```python
from build123d import *

# Parameters (mm, degrees)
BOSS_EXTRUDE1_DEPTH            = 4
CBORE_FOR_M3_SHCS2_D           = 3.4
CBORE_FOR_M3_SHCS2_CBORE_D     = 6.5
CBORE_FOR_M3_SHCS2_CBORE_DEPTH = 3
M5X0_8_TAPPED_HOLE1_D          = 4.2
M5X0_8_TAPPED_HOLE2_D          = 4.2
SKETCH8_W                      = 20
SKETCH8_H                      = 10
CUT_EXTRUDE1_DEPTH             = 5


with BuildPart() as part:
    # Sketch1 → Boss-Extrude1 (new body, symmetric)
    with BuildSketch(Plane.XY):
        with BuildLine():
            Line((-34.5, 0), (-49.5, 0))
            Line((-49.5, 0), (-49.5, 60))
            Line((-49.5, 60), (49.5, 60))
            Line((49.5, 60), (49.5, 0))
            Line((49.5, 0), (34.5, 0))
            Line((34.5, 0), (34.5, 47.5))
            ThreePointArc((34.5, 47.5), (33.767766953, 49.267766953), (32, 50))
            Line((32, 50), (-32, 50))
            ThreePointArc((-32, 50), (-33.767766953, 49.267766953), (-34.5, 47.5))
            Line((-34.5, 47.5), (-34.5, 0))
        make_face()
    extrude(amount=BOSS_EXTRUDE1_DEPTH, both=True)

    # CBORE for M3 SHCS2 (through all)
    with Locations(Plane.XY.offset(4)):
        with Locations((-42, 40), (-42, 20)):
            cbore_for_m3_shcs2 = CounterBoreHole(CBORE_FOR_M3_SHCS2_D / 2, CBORE_FOR_M3_SHCS2_CBORE_D / 2, CBORE_FOR_M3_SHCS2_CBORE_DEPTH)

    # M5x0.8 Tapped Hole1 (through all)
    with Locations(Plane.XY.offset(4)):
        with Locations((-42, 10), (-42, 50)):
            m5x0_8_tapped_hole1 = Hole(M5X0_8_TAPPED_HOLE1_D / 2)

    # M5x0.8 Tapped Hole2 (through all)
    with Locations(Plane(origin=(0, 60, 0), x_dir=(1, 0, 0), z_dir=(0, 1, 0))):
        with Locations((-28.5, 0)):
            m5x0_8_tapped_hole2 = Hole(M5X0_8_TAPPED_HOLE2_D / 2)

    # Mirror1: CBORE for M3 SHCS2, M5x0.8 Tapped Hole1, M5x0.8 Tapped Hole2 across plane
    add(cbore_for_m3_shcs2.mirror(Plane(origin=(0, 0, 0), x_dir=(0, 0, 1), z_dir=(1, 0, 0))), mode=Mode.SUBTRACT)
    add(m5x0_8_tapped_hole1.mirror(Plane(origin=(0, 0, 0), x_dir=(0, 0, 1), z_dir=(1, 0, 0))), mode=Mode.SUBTRACT)
    add(m5x0_8_tapped_hole2.mirror(Plane(origin=(0, 0, 0), x_dir=(0, 0, 1), z_dir=(1, 0, 0))), mode=Mode.SUBTRACT)

    # Sketch8 → Cut-Extrude1 (cut)
    with BuildSketch(Plane.XY.offset(4)):
        with Locations((0, 55)):
            Rectangle(SKETCH8_W, SKETCH8_H)
    extrude(amount=-CUT_EXTRUDE1_DEPTH, mode=Mode.SUBTRACT)


solid = part.part
```
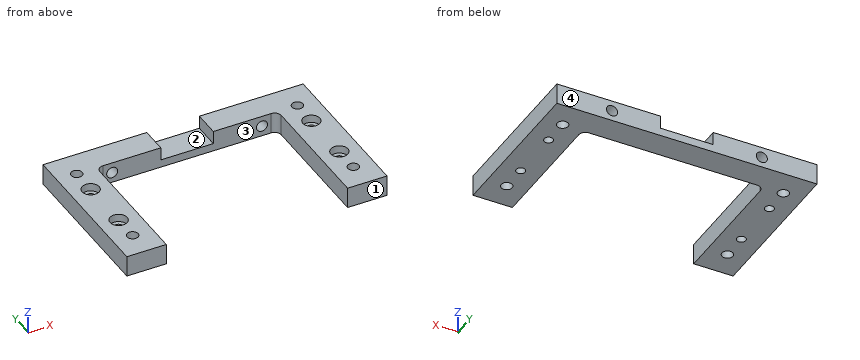
Here's how the part is built. I have some questions about the finished solid (model axes, mm). Face numbers are marked on the shaded views. A direction names the side the tool comes from. Coordinates: 2 decimals unless noted, no trailing zeros. Loops run counter-clockwise (first coordinate to the right, second up) from the corner with the lowest first, then second, coordinate; pieces in that order, holes last. Notation, with made-up numbers: M 28,25 L 46,25 A12 cw 46,32 Z; hole C 87,1 d6. An arc over 180 degrees is marked long. One line per item, written item: value.
1. Imagine slicing it at B-B (x = -42). List the corners of the cut face in (y, z) for me, and give its area (3 significant figures).
Geometry says:
outline: M 0,-4 L 7.9,-4 L 7.9,4 L 0,4 Z; M 12.1,-4 L 18.3,-4 L 18.3,1 L 16.75,1 L 16.75,4 L 12.1,4 Z; M 21.7,-4 L 38.3,-4 L 38.3,1 L 36.75,1 L 36.75,4 L 23.25,4 L 23.25,1 L 21.7,1 Z; M 41.7,-4 L 47.9,-4 L 47.9,4 L 43.25,4 L 43.25,1 L 41.7,1 Z; M 52.1,-4 L 60,-4 L 60,4 L 52.1,4 Z
area: 340 mm2
2. Imagine slicing it at C-C (y = 44.5). List the corners of the cut face in (x, z) for me, and give its area (3 significant figures).
Geometry says:
outline: M -49.5,-4 L -34.5,-4 L -34.5,4 L -49.5,4 Z; M 34.5,-4 L 49.5,-4 L 49.5,4 L 34.5,4 Z
area: 240 mm2
3. Thinking about a two-plate mould opening in X: for the marked faces 3 and 4, which applies, +X half, -X half, draft (parallel to the pull), parting line (faces both ways), or undercut?
Geometry says:
face 3: undercut
face 4: draft
4. Please list where these lines run through material, in increasing order: probe 1 along Y at (x, z) = (-42, 1.5); probe 2 along Y at (x, z) = (42, -0.9); probe 3 along X at (y, z) = (7, 1.75).
Geometry says:
probe 1: y = 0 to 7.9, 12.1 to 16.75, 23.25 to 36.75, 43.25 to 47.9, 52.1 to 60
probe 2: y = 0 to 7.9, 12.1 to 18.3, 21.7 to 38.3, 41.7 to 47.9, 52.1 to 60
probe 3: x = -49.5 to -34.5, 34.5 to 49.5
5. Imagine slicing it at A-A (y = 20). List the corners of the cut face in (x, z) for me.
Geometry says:
outline: M -49.5,-4 L -43.7,-4 L -43.7,1 L -45.25,1 L -45.25,4 L -49.5,4 Z; M -40.3,-4 L -34.5,-4 L -34.5,4 L -38.75,4 L -38.75,1 L -40.3,1 Z; M 34.5,-4 L 40.3,-4 L 40.3,1 L 38.75,1 L 38.75,4 L 34.5,4 Z; M 43.7,-4 L 49.5,-4 L 49.5,4 L 45.25,4 L 45.25,1 L 43.7,1 Z
6. On a 3-axis mill with a long thin cutter (end or side, diameter ignored), from which of +Z, -Z, +X, -X, +Y, -Y can I reach the whole of each face in a straight line? I mean the marked faces 1 and 2. Say none if no direction works.
Geometry says:
face 1: +Z, -Z, +X, -X, -Y
face 2: +Z, +Y, -Y
7. Imagine slicing it at D-D (x = -28.5). List the corners of the cut face in (y, z) for me.
Geometry says:
outline: M 50,-4 L 60,-4 L 60,-2.1 L 50,-2.1 Z; M 50,2.1 L 60,2.1 L 60,4 L 50,4 Z
8. Will these pins go through, and if not, where does the flat tip stop? pin 1 Ø5.5 at (x, y) = (42, 40) entering from +Z; pin 2 Ø11 at (x, y) = (0, 53) entering from +Z.
Geometry says:
pin 1: stops at z = 1
pin 2: stops at z = -1
